from build123d import *

# Parameters (mm, degrees)
BOSS_EXTRUDE1_START = -38.1
SKETCH1_R           = 3.968749999
SKETCH1_R_2         = 3.175
SKETCH1_R_3         = 3.174999999
BOSS_EXTRUDE1_DEPTH = 6.35
FILLET1_R           = 6.35


with BuildPart() as part:
    # Sketch1 → Boss-Extrude1 (new body)
    with BuildSketch(Plane(origin=(0, 0, 0), x_dir=(0, 0, -1), z_dir=(1, 0, 0)).offset(BOSS_EXTRUDE1_START)):
        with BuildLine():
            Line((23.324046982, 737.356140976), (23.324046982, 788.156140976))
            Line((23.324046982, 788.156140976), (76.2, 788.156140976))
            Line((76.2, 788.156140976), (165.505551403, 732.749973094))
            ThreePointArc((165.505551403, 732.749973094), (169.225626516, 720.873230423), (158.021191738, 715.455055766))
            Line((158.021191738, 715.455055766), (76.2, 737.356140976))
            Line((76.2, 737.356140976), (23.324046982, 737.356140976))
        make_face()
        with Locations((160.484046982, 724.656140976)):
            Circle(SKETCH1_R, mode=Mode.SUBTRACT)
        with Locations((62.346011746, 750.056140976)):
            Circle(SKETCH1_R_2, mode=Mode.SUBTRACT)
        with Locations((34.638035237, 750.056140976)):
            Circle(SKETCH1_R_3, mode=Mode.SUBTRACT)
        with Locations((34.638035237, 775.456140976)):
            Circle(SKETCH1_R_3, mode=Mode.SUBTRACT)
        with Locations((62.346011746, 775.456140976)):
            Circle(SKETCH1_R_2, mode=Mode.SUBTRACT)
    extrude(amount=-BOSS_EXTRUDE1_DEPTH)

    # Fillet1
    fillet1_edges = [part.edges().sort_by_distance(p)[0] for p in [
        (-41.275, 788.156140976, -76.2),
        (-41.275, 788.156140976, -23.324046982),
        (-41.275, 737.356140976, -23.324046982),
        (-41.275, 737.356140976, -76.2),
    ]]
    fillet(fillet1_edges, radius=FILLET1_R)


solid = part.part
Here's how the part is built. I have some questions about the finished solid (model axes, mm). A direction names the side the tool comes from. Coordinates: 2 decimals unless noted, no trailing zeros. Order: outer loops, then holes, each group sorted by start corner. A loop starts at its lowest first (then second) coordinate and runs counter-clockwise, first axis right, second up. Notation, with made-up numbers: (81.25, -24.5) -> (109.25, -24.5) arc R26 ccw to (109.25, 0.5) -> close; hole circle Ø2 at (-29.75, 37). An arc over 180 degrees is marked (long way). Answer in a Markdown table with one row per item.
(1) I want a section at C-C on x = -41. Count the separate pieces of the cut face and the enclosed holes in it, then the cut area to 3 significant figures.
Answer key:
| item | result |
|---|---|
| separate pieces | 1 |
| enclosed holes | 5 |
| area | 5,670 mm^2 |
(2) Please list where these lines run through material, in increasing order: probe 1 along Z at (x, y) = (-39.25, 749.5); probe 2 along Z at (x, y) = (-40.5, 778); probe 3 along Y at (x, z) = (-43, -64.5).
Answer key:
| item | result |
|---|---|
| probe 1 | -138.51 to -65.47, -59.22 to -37.76, -31.51 to -23.32 |
| probe 2 | -92.57 to -64.25, -60.45 to -36.54, -32.74 to -23.32 |
| probe 3 | 737.36 to 747.72, 752.39 to 773.12, 777.79 to 788.16 |
(3) I want a section at D-D on y = 780. List the corners of the cut face in (x, z) for me, then the cut area to 3 significant figures.
Answer key:
| item | result |
|---|---|
| outline | (-44.45, -89.35) -> (-38.1, -89.35) -> (-38.1, -23.32) -> (-44.45, -23.32) -> close |
| area | 419 mm^2 |
(4) I want a section at A-A on y = 723. List the corners of the cut face in (x, z) for me.
Answer key:
| item | result |
|---|---|
| outline | (-44.45, -169.86) -> (-38.1, -169.86) -> (-38.1, -164.09) -> (-44.45, -164.09) -> close; (-44.45, -156.88) -> (-38.1, -156.88) -> (-38.1, -129.83) -> (-44.45, -129.83) -> close |
(5) On a 3-axis mill with a long thin cutter (end or side, diameter ignored), from which of +Z, -Z, +X, -X, +Y, -Y can I reach the whole of each face in a straight line? I mean faces 1 (the face through (-41.2, 778.6, -34.2)), 2 (the face through (-41, 737.356, -53)). Say none if no direction works.
Answer key:
| item | result |
|---|---|
| face 1 | +X, -X |
| face 2 | +Z, +X, -X, -Y |
(6) Thinking about a two-plate mould opening in Y: for faces 3 (the face through (-41.231, 726.146, -118.081)), 4 (the face through (-41.23, 728.59, -159.97)), 5 (the face through (-41.231, 760.357, -121.007)), which applies, +Y half, -Y half, draft (parallel to the pull), parting line (faces both ways), or undercut?
Answer key:
| item | result |
|---|---|
| face 3 | -Y half |
| face 4 | undercut |
| face 5 | +Y half |
(7) I want a section at B-B on z = -34.5. List the corners of the cut face in (x, y) for me, then the cut area to 3 significant figures.
Answer key:
| item | result |
|---|---|
| outline | (-44.45, 737.36) -> (-38.1, 737.36) -> (-38.1, 746.88) -> (-44.45, 746.88) -> close; (-44.45, 753.23) -> (-38.1, 753.23) -> (-38.1, 772.28) -> (-44.45, 772.28) -> close; (-44.45, 778.63) -> (-38.1, 778.63) -> (-38.1, 788.16) -> (-44.45, 788.16) -> close |
| area | 242 mm^2 |
(8) Will these pins go through, and if not, where does the flat tip stop? pin 1 Ø3 at (x, y) = (-39.5, 723) entering from -Z; pin 2 Ø5.5 at (y, z) = (775.46, -62.35) entering from -X; pin 3 Ø3 at (x, z) = (-42.5, -49.5) entering from -Y.
Answer key:
| item | result |
|---|---|
| pin 1 | z = -170.01 |
| pin 2 | through |
| pin 3 | y = 737.36 |
